Input: part model. Units: mm. Frame: model coordinates. Coordinates: 2 decimals unless noted, no trailing zeros. Loops run counter-clockwise (first coordinate to the right, second up) from the corner with the lowest first, then second, coordinate; pieces in that order, holes last. Notation, with made-up numbers: M -24,37.25 L 4,37.25 A26 cw 4,74.25 Z; hole C 86,47 d3. An arc over 180 degrees is marked long. Use a Markdown table: item, result. Add a question column.
1. Section A-A on z = -8. Output: boundary loops of the cut face in (x, y) (3 decimals).
2. Section C-C on x = -4.5. Output: boundary loops of the cut face in (y, z) (3 decimals).
3. Pin query (flat end, axial travel): pin 1 (6 mm diameter, centred on x = -4, z = -11, fed in from +Y). Return the tip coordinate at first contact, or that it passes through.
4. Line query: L1, parallel to X at y = -177, z = 8 (3 decimals). Output: solid intervals per line, ascending. Write a range as [from, to].
5. Section B-B on y = -207. Output: boundary loops of the cut face in (x, z) (3 decimals), then the cut area to 3 significant figures.
```python
from build123d import *

# Parameters (mm, degrees)
SKETCH_W       = 31.75
SKETCH_H       = 31.75
SKETCH_W_2     = 26.2128
SKETCH_H_2     = 26.2128
PAD_DEPTH      = 304.8
PAD_DEPTH_BACK = 304.8
POCKET_DEPTH   = 31.75


with BuildPart() as part:
    # Sketch → Pad (new body, two sides)
    with BuildSketch(Plane.XZ) as pad_sk:
        Rectangle(SKETCH_W, SKETCH_H)
        Rectangle(SKETCH_W_2, SKETCH_H_2, mode=Mode.SUBTRACT)
    extrude(amount=PAD_DEPTH)
    extrude(pad_sk.sketch, amount=-PAD_DEPTH_BACK)

    # Sketch001 → Pocket (cut)
    with BuildSketch(Plane(origin=(0, 0, 15.875), x_dir=(-1, 0, 0), z_dir=(0, 0, 1))):
        Polygon((-15.875, -304.8), (15.875, -304.8), (15.875, -273.05), align=None)
    pocket = extrude(amount=-POCKET_DEPTH, mode=Mode.SUBTRACT)

    # Mirrored: Pocket across Sketch001 H_Axis
    add(pocket.mirror(Plane(origin=(0, 0, 15.875), x_dir=(0, 0, 1), z_dir=(0, -1, 0))), mode=Mode.SUBTRACT)


solid = part.part
```
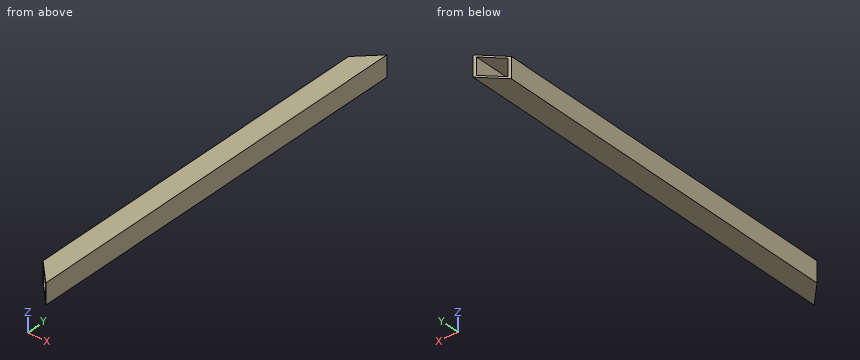
Answers below:
| question | item | result |
|---|---|---|
| 1 | outline | M -15.875,-273.05 L -13.106,-275.819 L -13.106,275.819 L -15.875,273.05 Z; M 13.106,-302.031 L 15.875,-304.8 L 15.875,304.8 L 13.106,302.031 Z |
| 2 | outline | M -284.425,-15.875 L 284.425,-15.875 L 284.425,-13.106 L -284.425,-13.106 Z; M -284.425,13.106 L 284.425,13.106 L 284.425,15.875 L -284.425,15.875 Z |
| 3 | pin 1 | stops at y = 287.06 |
| 4 | L1 | x = [-15.875, -13.106], [13.106, 15.875] |
| 5 | outline | M -15.875,-15.875 L 15.875,-15.875 L 15.875,15.875 L -15.875,15.875 Z; hole M -13.106,-13.106 L 13.106,-13.106 L 13.106,13.106 L -13.106,13.106 Z |
| 5 | area | 321 mm² |
